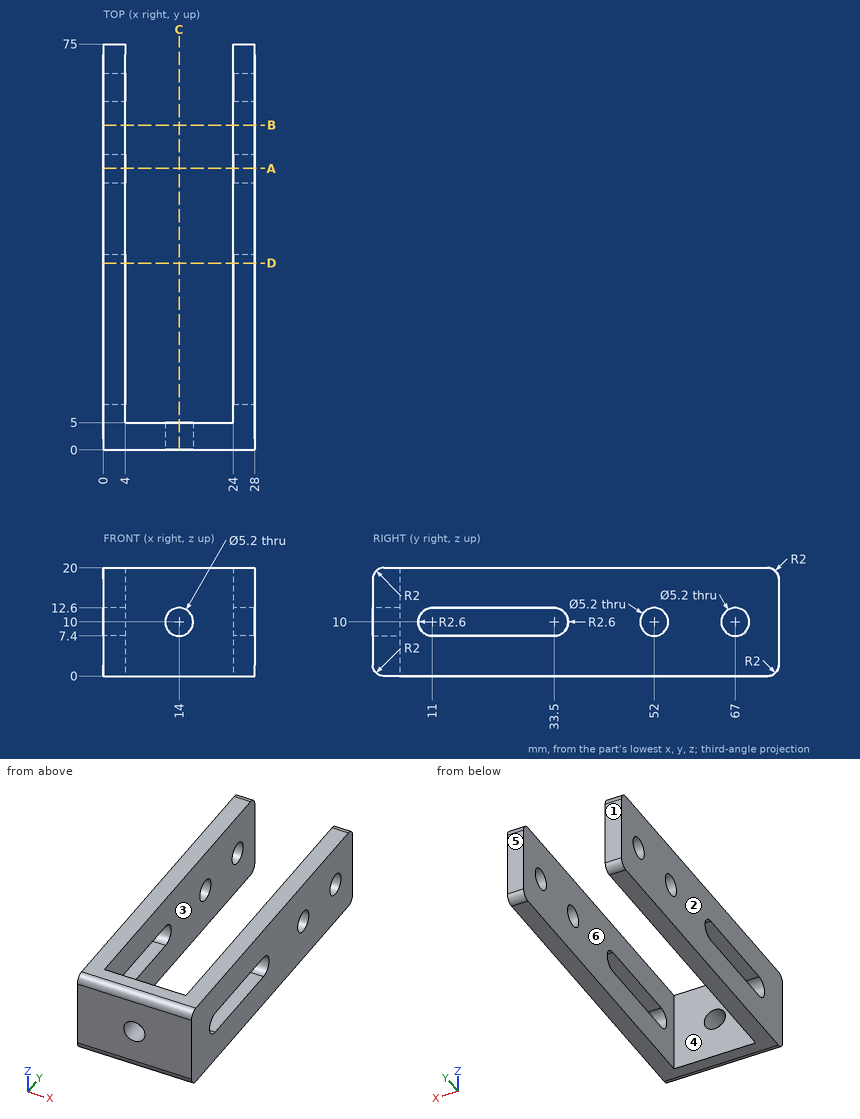
Geometry check sheet. Reference: drawing and pictorial views, mm from the part's lowest x, y, z. A direction names the side the tool comes from. Coordinates: 2 decimals unless noted, no trailing zeros. Loops run counter-clockwise (first coordinate to the right, second up) from the corner with the lowest first, then second, coordinate; pieces in that order, holes last. Notation, with made-up numbers: (69.25, 31) -> (123.25, 31) arc R22 cw to (123.25, 42) -> close; hole circle Ø2 at (-8, 45). An arc over 180 degrees is marked (long way). Write item = value, one per line. Start each with the question number.
1. Draft check along X on the marked faces 1, 2, 3 and 4. Enter one of: released by +X, released by -X, zero draft, split by the parting line, or undercut.
2. Section check D-D on y = 34.5. Record the cut outline in (x, z), then the cut area to 3 significant figures.
3. Section check A-A on y = 52. Record the cut outline in (x, z), then the cut area to 3 significant figures.
4. Material ranges on line 1 (Y direction, x = 2.7, z = 10); line 2 (X direction, y = 10.5, z = 13.5); line 3 (X direction, y = 1.45, z = 10), recorded low to high.
5. Tool access check on the marked faces 5 and 6. Record the directions out of +Z, -Z, +X, -X, +Y, -Y that give a thin tool (end or side, any length) a straight path to the whole face; none if there is none.
6. Section check B-B on y = 60. Record the cut outline in (x, z).
7. Depth check by flat-ended pin: P1, Ø6, axis at x = 14, z = 10, coming from the +Y side. Enter the tip coordinate at first touch or a pass-through.
8. Section check C-C on x = 14. Record the cut outline in (y, z), then the cut area to 3 significant figures.
Responses:
q1.face_1 = zero draft
q1.face_2 = released by -X
q1.face_3 = undercut
q1.face_4 = undercut
q2.outline = (0, 0) -> (4, 0) -> (4, 7.6) -> (0, 7.6) -> close; (0, 12.4) -> (4, 12.4) -> (4, 20) -> (0, 20) -> close; (24, 0) -> (28, 0) -> (28, 7.6) -> (24, 7.6) -> close; (24, 12.4) -> (28, 12.4) -> (28, 20) -> (24, 20) -> close
q2.area = 122 mm2
q3.outline = (0, 0) -> (4, 0) -> (4, 7.4) -> (0, 7.4) -> close; (0, 12.6) -> (4, 12.6) -> (4, 20) -> (0, 20) -> close; (24, 0) -> (28, 0) -> (28, 7.4) -> (24, 7.4) -> close; (24, 12.6) -> (28, 12.6) -> (28, 20) -> (24, 20) -> close
q3.area = 118 mm2
q4.line_1 = 0 to 8.4, 36.1 to 49.4, 54.6 to 64.4, 69.6 to 75
q4.line_2 = 0 to 4, 24 to 28
q4.line_3 = 0 to 11.4, 16.6 to 28
q5.face_5 = +Z, -Z, +X, -X, +Y
q5.face_6 = +Z, -Z, +Y
q6.outline = (0, 0) -> (4, 0) -> (4, 20) -> (0, 20) -> close; (24, 0) -> (28, 0) -> (28, 20) -> (24, 20) -> close
q7.P1 = 5
q8.outline = (0, 2) arc R2 ccw to (2, 0) -> (5, 0) -> (5, 7.4) -> (0, 7.4) -> close; (0, 12.6) -> (5, 12.6) -> (5, 20) -> (2, 20) arc R2 ccw to (0, 18) -> close
q8.area = 72.3 mm2
